Check sheet for the modelled part. Datum: model origin and axes. Units: mm. A direction names the side the tool comes from. Round coordinates to 2 decimals unless told otherwise and drop trailing zeros. Loops run counter-clockwise (first coordinate to the right, second up) from the corner with the lowest first, then second, coordinate; pieces in that order, holes last. Notation, with made-up numbers: (22, -12.75) -> (49, -12.75) arc R11 ccw to (49, -7.75) -> close; hole circle Ø11 at (-7.5, 11). An arc over 180 degrees is marked (long way). One line per question, with ' | ' between items.
```python
from build123d import *

# Parameters (mm, degrees)
F0_R     = 47.9922028916
F0_R_2   = 30.5721704199
F1_DEPTH = 418.592
F3_DEPTH = 68.58
F5_DEPTH = 78.74
F6_R     = 30.5721704199
F6_R_2   = 24.281009231
F7_DEPTH = 495.3


with BuildPart() as f1:
    # F0 (on Top) → F1 (new body)
    with BuildSketch(Plane.XY):
        Circle(F0_R)
        Circle(F0_R_2, mode=Mode.SUBTRACT)
    extrude(amount=-F1_DEPTH)

    # F2 (on face) → F3 (join)
    with BuildSketch(Plane.XY):
        with BuildLine():
            Line((-47.9922028916, 228.3145189285), (-47.9922028916, 0))
            Line((-47.9922028916, 0), (47.6234853268, 0))
            Line((47.6234853268, 0), (47.6234853268, 228.3145189285))
            ThreePointArc((47.6234853268, 228.3145189285), (-0.1843587824, 180.5066748193), (-47.9922028916, 228.3145189285))
        make_face()
        with BuildLine():
            ThreePointArc((47.6234853268, 228.3145189285), (-0.1843587824, 276.1223630377), (-47.9922028916, 228.3145189285))
            Line((-47.9922028916, 228.3145189285), (-25.5504139221, 228.3145189285))
            ThreePointArc((-25.5504139221, 228.3145189285), (-0.1843587824, 253.6805740682), (25.1816963573, 228.3145189285))
            Line((25.1816963573, 228.3145189285), (47.6234853268, 228.3145189285))
        make_face()
        with BuildLine():
            Line((-25.5504139221, 228.3145189285), (-47.9922028916, 228.3145189285))
            ThreePointArc((-47.9922028916, 228.3145189285), (-0.1843587824, 180.5066748193), (47.6234853268, 228.3145189285))
            Line((47.6234853268, 228.3145189285), (25.1816963573, 228.3145189285))
            ThreePointArc((25.1816963573, 228.3145189285), (-0.1843587824, 202.9484637888), (-25.5504139221, 228.3145189285))
        make_face()
    extrude(amount=-F3_DEPTH)

    # F4 (on face) → F5 (join)
    with BuildSketch(Plane(origin=(0, 0, -418.592), x_dir=(1, 0, 0), z_dir=(0, 0, -1))):
        with BuildLine():
            Line((47.9922028916, -243.720613562), (47.9922028916, 0))
            Line((47.9922028916, 0), (-48.7415492535, 0))
            Line((-48.7415492535, 0), (-48.7415492535, -252.2345483303))
            ThreePointArc((-48.7415492535, -252.2345483303), (-4.2734238383, -203.6806970688), (47.9922028916, -243.720613562))
        make_face()
        with BuildLine():
            ThreePointArc((48.7415492535, -252.2345483303), (48.5538512615, -247.961124492), (47.9922028916, -243.720613562))
            Line((47.9922028916, -243.720613562), (47.9922028916, -252.2345483303))
            Line((47.9922028916, -252.2345483303), (-48.7415492535, -252.2345483303))
            ThreePointArc((-48.7415492535, -252.2345483303), (0, -300.9760975838), (48.7415492535, -252.2345483303))
        make_face()
        with BuildLine():
            Line((47.9922028916, -252.2345483303), (47.9922028916, -243.720613562))
            ThreePointArc((47.9922028916, -243.720613562), (-4.2734238383, -203.6806970688), (-48.7415492535, -252.2345483303))
            Line((-48.7415492535, -252.2345483303), (47.9922028916, -252.2345483303))
        make_face()
    extrude(amount=-F5_DEPTH)

    # F6 (on face) → F7 (cut)
    with BuildSketch(Plane.XY):
        Circle(F6_R)
        with Locations((-0.1843587824, 228.3145189285)):
            Circle(F6_R_2)
    extrude(amount=-F7_DEPTH, mode=Mode.SUBTRACT)


solid = f1.part
```
(1) Sectioned sample at B-B, the plane z = -61.5. Record the cut outline in (x, y).
Answer:
outline: (-47.99, 0) arc R47.99 ccw (long way) to (47.62, 5.94) -> (47.62, 228.31) arc R47.81 ccw to (-47.99, 228.31) -> close; hole circle Ø61.14 at (0, 0); hole circle Ø50.73 at (-0.18, 228.31)
(2) Sectioned sample at C-C, the plane x = 0. Record the cut outline in (y, z), and give its area (3 significant figures).
Answer:
outline: (-47.99, -418.59) -> (-30.57, -418.59) -> (-30.57, 0) -> (-47.99, 0) -> close; (30.57, -418.59) -> (204.03, -418.59) -> (204.03, -339.85) -> (47.99, -339.85) -> (47.99, -68.58) -> (202.95, -68.58) -> (202.95, 0) -> (30.57, 0) -> close; (252.59, -418.59) -> (300.98, -418.59) -> (300.98, -339.85) -> (252.59, -339.85) -> close; (253.68, -68.58) -> (276.12, -68.58) -> (276.12, 0) -> (253.68, 0) -> close | area: 42,800 mm2
(3) Sectioned sample at A-A, the plane y = 234. Record the cut outline in (x, z).
Answer:
outline: (-48.74, -418.59) -> (-23.79, -418.59) -> (-23.79, -339.85) -> (-48.74, -339.85) -> close; (-47.65, -68.58) -> (-24.91, -68.58) -> (-24.91, 0) -> (-47.65, 0) -> close; (23.42, -418.59) -> (47.99, -418.59) -> (47.99, -339.85) -> (23.42, -339.85) -> close; (24.54, -68.58) -> (47.28, -68.58) -> (47.28, 0) -> (24.54, 0) -> close
(4) Go/stop test with flat-tipped pins: pin 1 (3 mm diameter, centred on x = -23, y = 222.5, fed in from +Z); pin 2 (20.5 mm diameter, centred on y = 149.5, z = -25.5, fed in from +X); pin 3 (1 mm diameter, centred on y = -5, z = -103.5, fed in from +X). Record where each tip stops, or that it passes through.
Answer:
pin 1: stops at z = -339.85 | pin 2: stops at x = 47.62 | pin 3: stops at x = 47.78
(5) Scan lines: probe 1 along Z at (x, y) = (6, 92); probe 2 along Y at (x, z) = (0, -301.5). Record each from-to range of solid material in increasing order.
Answer:
probe 1: z = -418.59 to -339.85, -68.58 to 0 | probe 2: y = -47.99 to -30.57, 30.57 to 47.99
(6) Sectioned sample at D-D, the plane z = -282. Record the cut outline in (x, y).
Answer:
outline: circle Ø95.98 at (0, 0); hole circle Ø61.14 at (0, 0)
(7) Set-up check for faces 4 (the face through (47.992, 124, -380)), 5 (the face through (0.87, 276.11, -33.81)), 6 (the face through (-10.4, -46.85, -206.37)), 7 (the face through (3.118, 253.465, -33.81)): record each of +Z, -Z, +X, -X, +Y, -Y from which the full face is reachable in a straight line by a thin tool's end or side.
Answer:
face 4: +Z, -Z, +X, -Y | face 5: +Z, +Y | face 6: none | face 7: +Z
(8) Mould release check, pull along X, two halves, no side actions. Record for faces 1 (the face through (47.623, 116, -34)), 2 (the face through (-3.35, 252.39, -378.67)), 3 (the face through (-47.992, 116, -34)): +X half, -X half, draft (parallel to the pull), parting line (faces both ways), or undercut.
Answer:
face 1: +X half | face 2: undercut | face 3: -X half
